from build123d import *

# Parameters (mm, degrees)
F0_W     = 44.45
F0_H     = 31.75
F0_W_2   = 6.35
F1_DEPTH = 6.35


with BuildPart() as f1:
    # F0 (on Front) → F1 (new body)
    with BuildSketch(Plane.XZ):
        with Locations((-50.8, 15.875)):
            Rectangle(F0_W, F0_H)
        with Locations((0, 15.875)):
            Rectangle(F0_W, F0_H)
        with Locations((50.8, 15.875)):
            Rectangle(F0_W, F0_H)
        with Locations((-50.8, -15.875)):
            Rectangle(F0_W, F0_H)
        with Locations((0, -15.875)):
            Rectangle(F0_W, F0_H)
        with Locations((50.8, -15.875)):
            Rectangle(F0_W, F0_H)
        with Locations((-76.2, -15.875)):
            Rectangle(F0_W_2, F0_H)
        with Locations((-25.4, -15.875)):
            Rectangle(F0_W_2, F0_H)
        with Locations((25.4, -15.875)):
            Rectangle(F0_W_2, F0_H)
        with Locations((76.2, -15.875)):
            Rectangle(F0_W_2, F0_H)
    extrude(amount=F1_DEPTH)


solid = f1.part
Can you work these out from the model? Positions are in its coordinate system, mm. A direction names the side the tool comes from. Coordinates: 2 decimals unless noted, no trailing zeros. Loops run counter-clockwise (first coordinate to the right, second up) from the corner with the lowest first, then second, coordinate; pieces in that order, holes last. Notation, with made-up numbers: (-8, -22.5) - (51, -22.5) arc R12 ccw to (51, -15.5) - close; hole circle Ø4 at (87, 87.5). An arc over 180 degrees is marked (long way). Put each result on its own line as item: value. Start each with the question number.
Item 1: If I drill on line 1 along X through (y, z) = (-2.75, 5) (3 decimals); line 2 along Z through (x, y) = (24, -1), over which ranges is the centre line in solid material (lowest first)?
Item 2: Which directions (+Z, -Z, +X, -X, +Y, -Y) give clear straight access to the entire face, cutting with the end or side of a thin tool? Please do faces 5 (the face through (-73.025, -3, 16)), 6 (the face through (-1, -3, -31.75)), 7 (the face through (-28.575, -3, 16)), 8 (the face through (76, -3, 0)).
Item 3: Suppose I cut it at A-A (z = 17). Please give me the cut outline in (x, y) (3 decimals).
Item 4: Suppose I cut it at B-B (y = -3.25). Please give me the cut outline in (x, z) (3 decimals), and give its area (3 significant figures).
Item 5: For pin 1 (1.9 mm diameter, centred on y = -2.5, z = 16.5, fed in from -X) (3 decimals), with a flat end and sliding along its axis, tell me the tip position at first contact or that it passes through.
Item 6: If we mould it in two halves opening along X, with no side actions, what happens to faces 1 (the face through (79.375, -3, -16)), 2 (the face through (28.575, -3, 16)), 3 (the face through (-1, -6.35, 0)), 4 (the face through (25, -3, 0))? For each: +X half, -X half, draft (parallel to the pull), parting line (faces both ways), or undercut.
Here are the results:
1. line 1: -73.025 to -28.575, -22.225 to 22.225, 28.575 to 73.025
1. line 2: -31.75 to 0
2. face 5: +Z, -X, +Y, -Y
2. face 6: -Z, +X, -X, +Y, -Y
2. face 7: +Z, +Y, -Y
2. face 8: +Z, +X, +Y, -Y
3. outline: (-73.025, -6.35) - (-28.575, -6.35) - (-28.575, 0) - (-73.025, 0) - close; (-22.225, -6.35) - (22.225, -6.35) - (22.225, 0) - (-22.225, 0) - close; (28.575, -6.35) - (73.025, -6.35) - (73.025, 0) - (28.575, 0) - close
4. outline: (-79.375, -31.75) - (79.375, -31.75) - (79.375, 0) - (73.025, 0) - (73.025, 31.75) - (28.575, 31.75) - (28.575, 0) - (22.225, 0) - (22.225, 31.75) - (-22.225, 31.75) - (-22.225, 0) - (-28.575, 0) - (-28.575, 31.75) - (-73.025, 31.75) - (-73.025, 0) - (-79.375, 0) - close
4. area: 9,270 mm²
5. pin 1: x = -73.025
6. face 1: +X half
6. face 2: undercut
6. face 3: draft
6. face 4: undercut
